```python
from build123d import *

# Parameters (mm, degrees)
SKETCH_1_R          = 1.6
EXTRUDE_1_DEPTH     = 8
SKETCH_2_R          = 3
CUT_EXTRUDE_1_DEPTH = 3
FILLET_1_R          = 10
EXTRUDE_START       = -18.399949
SKETCH_3_R          = 1.6
EXTRUDE_2_DEPTH     = 18.399949
SKETCH_5_R          = 3
CUT_EXTRUDE_2_DEPTH = 3
FILLET_2_R          = 10


with BuildPart() as part:
    # 草图1 → 凸台-拉伸1 (new body)
    with BuildSketch(Plane.XY):
        Polygon((10, 57.5), (10, 27.5), (-10, 27.5), (-10, 77.5), (40, 77.5), (40, 57.5), align=None)
        with Locations((32, 67.5)):
            Circle(SKETCH_1_R, mode=Mode.SUBTRACT)
        with Locations((18, 67.5)):
            Circle(SKETCH_1_R, mode=Mode.SUBTRACT)
        with Locations((0, 62.5)):
            Circle(SKETCH_1_R, mode=Mode.SUBTRACT)
        with Locations((0, 42.5)):
            Circle(SKETCH_1_R, mode=Mode.SUBTRACT)
    extrude(amount=EXTRUDE_1_DEPTH)

    # 草图2 → 切除-拉伸1 (cut)
    with BuildSketch(Plane.XY.offset(8)):
        with Locations((32, 67.5)):
            Circle(SKETCH_2_R)
        with Locations((18, 67.5)):
            Circle(SKETCH_2_R)
        with Locations((0, 62.5)):
            Circle(SKETCH_2_R)
        with Locations((0, 42.5)):
            Circle(SKETCH_2_R)
    extrude(amount=-CUT_EXTRUDE_1_DEPTH, mode=Mode.SUBTRACT)

    # 圆角1
    fillet_1_edges = [part.edges().sort_by_distance(p)[0] for p in [
        (-10, 77.5, 4),
        (10, 57.5, 4),
    ]]
    fillet(fillet_1_edges, radius=FILLET_1_R)

    # 草图3 → 凸台-拉伸2 (add)
    with BuildSketch(Plane.XY.offset(8).offset(EXTRUDE_START)):
        with BuildLine():
            Line((40, 27.5), (40, 57.5))
            Line((40, 57.5), (20, 57.5))
            ThreePointArc((20, 57.5), (12.939135643, 54.581256565), (10.000041584, 47.528838907))
            ThreePointArc((10.000041584, 47.528838907), (10.000010396, 47.514419468), (10, 47.5))
            Line((10, 47.5), (10, 27.5))
            Line((10, 27.5), (40, 27.5))
        make_face()
        with Locations((20, 47.528839027)):
            Circle(SKETCH_3_R, mode=Mode.SUBTRACT)
    extrude(amount=EXTRUDE_2_DEPTH)

    # 草图5 → 切除-拉伸2 (cut)
    with BuildSketch(Plane.XY.offset(8)):
        with Locations((20, 47.528839027)):
            Circle(SKETCH_5_R)
    extrude(amount=-CUT_EXTRUDE_2_DEPTH, mode=Mode.SUBTRACT)

    # 圆角2
    fillet_2_edges = [part.edges().sort_by_distance(p)[0] for p in [
        (40, 57.5, -5.1999745),
        (10, 27.5, -5.1999745),
        (40, 27.5, -1.1999745),
    ]]
    fillet(fillet_2_edges, radius=FILLET_2_R)


solid = part.part
```
Geometry check sheet. Reference: the model listing, model coordinates, mm. A direction names the side the tool comes from. Round coordinates to 2 decimals unless told otherwise and drop trailing zeros. Order: outer loops, then holes, each group sorted by start corner. A loop starts at its lowest first (then second) coordinate and runs counter-clockwise, first axis right, second up. Notation, with made-up numbers: (-0.5, 31) - (25.5, 31) arc R21 ccw to (25.5, 58) - close; hole circle Ø1 at (12.25, 3.5). An arc over 180 degrees is marked (long way). Use a Markdown table: item, result. Add a question column.
1) Thickness scan on line 1 along Y through (x, z) = (0, 1.6); line 2 along Y through (x, z) = (20, -6); line 3 along Y through (x, z) = (20, 6.25). Record the ranges inside material, lowest first.
2) Section check A-A (y = 62.5). Record the cut outline in (x, z), then the cut area to 3 significant figures.
3) Set-up check for faces 4 (the cylindrical face through (17.35, 64.57, 6.52)), 5 (the flat face through (10, 43, -5)), 6 (the cylindrical face through (13.02, 54.66, -5.27)): record each of +Z, -Z, +X, -X, +Y, -Y from which the full face is reachable in a straight line by a thin tool's end or side.
4) Section check C-C (x = 32). Record the cut outline in (y, z), then the cut area to 3 significant figures.
5) Gauge pin test, flat ends, axial feed: P1, Ø5, axis at x = 0, y = 42.5, coming from the -Z side; P2, Ø5.5, axis at x = 0, y = 62.5, coming from the +Z side; P3, Ø8, axis at x = 25.5, z = -4.5, coming from the +Y side. Record the tip position at first contact, or that the pin passes through.
6) Mould release check, pull along Y, two halves, no side actions. Record for faces 1 (the cylindrical face through (-7.15, 74.49, 4.06)), 2 (the flat face through (10, 58, 0)), 3 (the cylindrical face through (19.35, 44.6, 6.52)): released by +Y, released by -Y, zero draft, split by the parting line, or undercut.
7) Section check B-B (z = 2). Record the cut outline in (x, y), then the cut area to 3 significant figures.
Established:
| question | item | result |
|---|---|---|
| 1 | line 1 | 27.5 to 40.9, 44.1 to 60.9, 64.1 to 77.5 |
| 1 | line 2 | 27.5 to 45.93, 49.13 to 57.5 |
| 1 | line 3 | 27.5 to 44.53, 50.53 to 65.26, 69.74 to 77.5 |
| 2 | outline | (-10, 0) - (-1.6, 0) - (-1.6, 5) - (-3, 5) - (-3, 8) - (-10, 8) - close; (1.6, 0) - (40, 0) - (40, 8) - (3, 8) - (3, 5) - (1.6, 5) - close |
| 2 | area | 366 mm2 |
| 3 | face 4 | +Z |
| 3 | face 5 | -Z, -X, +Y, -Y |
| 3 | face 6 | -Z, -X, +Y |
| 4 | outline | (27.7, -10.4) - (57.3, -10.4) - (57.3, 0) - (65.9, 0) - (65.9, 5) - (64.5, 5) - (64.5, 8) - (27.7, 8) - close; (69.1, 0) - (77.5, 0) - (77.5, 8) - (70.5, 8) - (70.5, 5) - (69.1, 5) - close |
| 4 | area | 672 mm2 |
| 5 | P1 | z = 0 |
| 5 | P2 | z = 5 |
| 5 | P3 | y = 57.5 |
| 6 | face 1 | released by +Y |
| 6 | face 2 | zero draft |
| 6 | face 3 | undercut |
| 7 | outline | (-10, 27.5) - (30, 27.5) arc R10 ccw to (40, 37.5) - (40, 77.5) - (0, 77.5) arc R10 ccw to (-10, 67.5) - close; hole circle Ø3.2 at (0, 42.5); hole circle Ø3.2 at (0, 62.5); hole circle Ø3.2 at (18, 67.5); hole circle Ø3.2 at (20, 47.53); hole circle Ø3.2 at (32, 67.5) |
| 7 | area | 2,420 mm2 |
